```python
from build123d import *

# Parameters (mm, degrees)
SKETCH1_W           = 20
SKETCH1_H           = 71.5
SKETCH1_R           = 2.5
BOSS_EXTRUDE1_DEPTH = 5
BOSS_EXTRUDE2_DEPTH = 20
CUT_EXTRUDE1_REACH  = 82.562
SKETCH3_R           = 3.5
SKETCH4_R           = 1.5
CUT_EXTRUDE2_DEPTH  = 10


with BuildPart() as part:
    # Sketch1 → Boss-Extrude1 (new, symmetric)
    with BuildSketch(Plane.XY):
        Rectangle(SKETCH1_W, SKETCH1_H)
        with Locations((0, 25.75)):
            Circle(SKETCH1_R, mode=Mode.SUBTRACT)
        with Locations((0, 10.75)):
            Circle(SKETCH1_R, mode=Mode.SUBTRACT)
    extrude(amount=BOSS_EXTRUDE1_DEPTH, both=True)

    # Sketch2 → Boss-Extrude2 (add, through all)
    with BuildSketch(Plane(origin=(10, 0, 0), x_dir=(0, 0, -1), z_dir=(1, 0, 0))):
        Polygon((5, 35.75), (5, -35.75), (76.5, -35.75), align=None)
    extrude(amount=-BOSS_EXTRUDE2_DEPTH)

    # Cut-Extrude1: up to this plane
    cut_extrude1_end = Plane(origin=(-10, -35.75, -76.5), z_dir=(0, 0.7071067811865439, -0.7071067811865512))
    # Sketch3 → Cut-Extrude1 (cut, up to the surface)
    with BuildSketch(Plane.XY.offset(-5), mode=Mode.PRIVATE) as cut_extrude1_sk1:
        with Locations((0, 25.75)):
            Circle(SKETCH3_R)
    cut_extrude1_tool1 = split(extrude(cut_extrude1_sk1.sketch, amount=-CUT_EXTRUDE1_REACH, mode=Mode.PRIVATE), bisect_by=cut_extrude1_end, keep=Keep.BOTH, mode=Mode.PRIVATE)
    add(cut_extrude1_tool1.solids().sort_by_distance((0, 25.75, -5))[0], mode=Mode.SUBTRACT)
    # Sketch3 → Cut-Extrude1 (cut, up to the surface)
    with BuildSketch(Plane.XY.offset(-5), mode=Mode.PRIVATE) as cut_extrude1_sk2:
        with Locations((0, 10.75)):
            Circle(SKETCH3_R)
    cut_extrude1_tool2 = split(extrude(cut_extrude1_sk2.sketch, amount=-CUT_EXTRUDE1_REACH, mode=Mode.PRIVATE), bisect_by=cut_extrude1_end, keep=Keep.BOTH, mode=Mode.PRIVATE)
    add(cut_extrude1_tool2.solids().sort_by_distance((0, 10.75, -5))[0], mode=Mode.SUBTRACT)

    # Sketch4 → Cut-Extrude2 (cut)
    with BuildSketch(Plane.XZ.offset(35.75)):
        with Locations(Location((0, -5, 0), (0, 0, 270))):
            Circle(SKETCH4_R)
        with Locations(Location((0, -45, 0), (0, 0, 270))):
            Circle(SKETCH4_R)
    extrude(amount=-CUT_EXTRUDE2_DEPTH, mode=Mode.SUBTRACT)


solid = part.part
```
CAD build for the part. Positions are in the model's coordinates, mm. A direction names the side the tool comes from. Round coordinates to 2 decimals unless told otherwise and drop trailing zeros. Loops run counter-clockwise (first coordinate to the right, second up) from the corner with the lowest first, then second, coordinate; pieces in that order, holes last. Notation, with made-up numbers: (78, 18.25) - (89, 18.25) arc R25 cw to (89, 41.25) - close; hole circle Ø11 at (15.25, 30). An arc over 180 degrees is marked (long way). Return JSON: item names as keys, results as strings. Group by question number.
Q1. Drill centre lines: line 1 along Y through (x, z) = (0, 1); line 2 along X through (y, z) = (25.75, -8.25); line 3 along Y through (x, z) = (-3.5, -66.5). Where is each one in solid material? Low to high. Write a range as [from, to].
Q2. Two-plate mould, pull along Y, no slides. Class faces 4 (the face through (1.5, 8.5, -5)), 5 (the face through (-0.33, 28.23, -0.07)), 6 (the face through (0.07, -30.82, -43.5)), 7 (the face through (0, -25.75, -5)): +Y half, -Y half, draft (parallel to the pull), parting line (faces both ways), or undercut.
Q3. Tool access for faces 1 (the face through (10, -8, -26)), 2 (the face through (-0.759, 7.333, -19.051)), 3 (the face through (0, -25.75, -45)): list every direction of +Z, -Z, +X, -X, +Y, -Y with a clear straight run to the whole face (end or side of a thin tool).
Q4. Band-saw the part on A-A on y = 10.75. Give the cut face in (x, z), plus the area to 3 significant figures.
Q5. Band-saw the part on D-D on z = -45. Give the cut face in (x, y).
Q6. Band-saw the part on B-B on x = 0. Give the cut face in (y, z), plus the area to 3 significant figures.
Q7. Band-saw the part on C-C on z = -2.5. Give the cut face in (x, y).
Q8. Flat gauge pins, fed straight in: pin 1 Ø3 at (x, y) = (0, 25.75) entering from +Z; pin 2 Ø1.5 at (x, z) = (0.5, -44.5) entering from -Y; pin 3 Ø6.5 at (x, y) = (0, 10.75) entering from -Z; pin 4 Ø3.5 at (x, y) = (1.5, 9.5) entering from -Z. Where does each tip first touch, or does it go through?
Solutions:
{
 "1": {"line 1": "y = [-35.75, 8.25], [13.25, 23.25], [28.25, 35.75]", "line 2": "x = [-10, -3.5], [3.5, 10]", "line 3": "y = [-35.75, -25.75]"},
 "2": {"face 4": "undercut", "face 5": "undercut", "face 6": "draft", "face 7": "-Y half"},
 "3": {"face 1": "+Z, -Z, +X, +Y, -Y", "face 2": "-Z", "face 3": "-Y"},
 "4": {"outline": "(-10, -30) - (-3.5, -30) - (-3.5, -5) - (-2.5, -5) - (-2.5, 5) - (-10, 5) - close; (2.5, -5) - (3.5, -5) - (3.5, -30) - (10, -30) - (10, 5) - (2.5, 5) - close", "area": "475 mm^2"},
 "5": {"outline": "(-10, -35.75) - (-1.5, -35.75) - (-1.5, -25.75) - (1.5, -25.75) - (1.5, -35.75) - (10, -35.75) - (10, -4.25) - (-10, -4.25) - close"},
 "6": {"outline": "(-35.75, -76.5) - (7.25, -33.5) - (7.25, -5) - (8.25, -5) - (8.25, 5) - (-35.75, 5) - (-35.75, -3.5) - (-25.75, -3.5) - (-25.75, -6.5) - (-35.75, -6.5) - (-35.75, -43.5) - (-25.75, -43.5) - (-25.75, -46.5) - (-35.75, -46.5) - close; (13.25, -5) - (14.25, -5) - (14.25, -26.5) - (22.25, -18.5) - (22.25, -5) - (23.25, -5) - (23.25, 5) - (13.25, 5) - close; (28.25, -5) - (29.25, -5) - (29.25, -11.5) - (35.75, -5) - (35.75, 5) - (28.25, 5) - close", "area": "2,870 mm^2"},
 "7": {"outline": "(-10, -35.75) - (10, -35.75) - (10, 35.75) - (-10, 35.75) - close; hole circle Ø5 at (0, 10.75); hole circle Ø5 at (0, 25.75)"},
 "8": {"pin 1": "passes through", "pin 2": "stops at y = -25.75", "pin 3": "stops at z = -5", "pin 4": "stops at z = -32.96"}
}
